The figure shows three views and two pictorial views of one solid part (mm, origin at its lowest corner). Answer the questions. A direction names the side the tool comes from. Give positions to 0.01 mm unless a question says otherwise; leave off trailing zeros. Order: outer loops, then holes, each group sorted by start corner. A loop starts at its lowest first (then second) coordinate and runs counter-clockwise, first axis right, second up. Notation, with made-up numbers: (-10, -5) - (1, -5) arc R34 ccw to (1, 29) - close; hole circle Ø11 at (39, 53). An arc over 180 degrees is marked (long way). Write item = value, one per line.
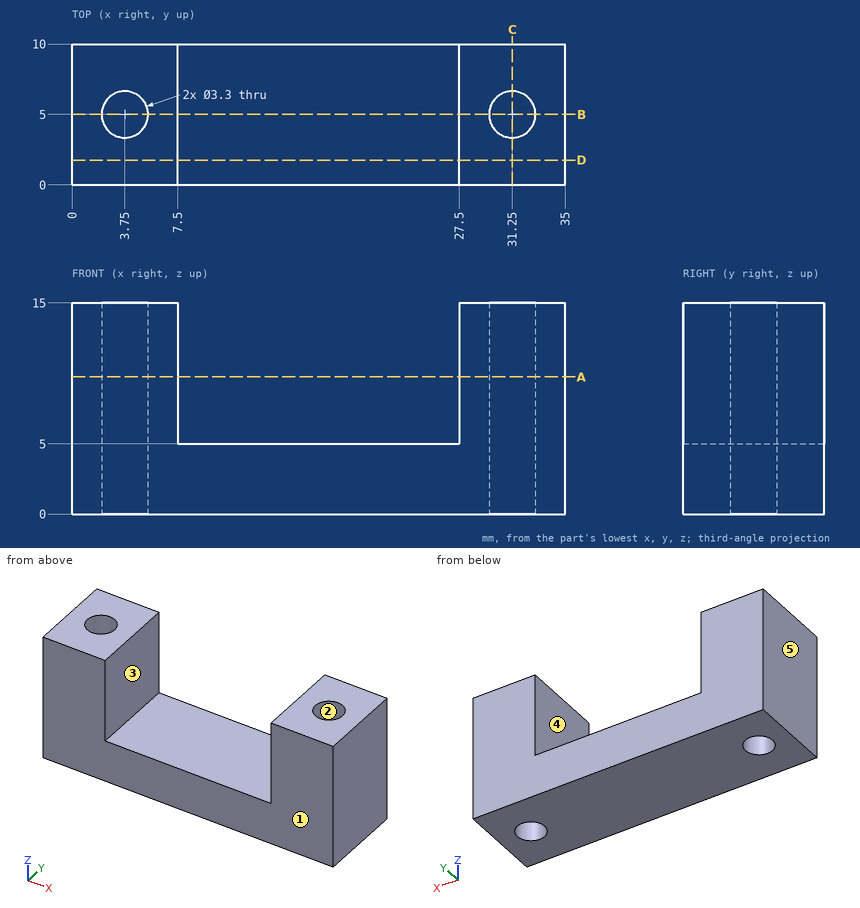
1. Determine the mould class of the marked faces 1, 2 and 3 for opening direction Y: +Y half, -Y half, draft (parallel to the pull), parting line (faces both ways), or undercut.
Recorded:
face_1 = -Y half
face_2 = undercut
face_3 = draft
2. Straight lines are drawn through the part: L1, parallel to Y at x = 31.25, z = 5.5; L2, parallel to X at y = 9, z = 9.25; L3, parallel to X at y = 5.25, z = 1.5. For each, find the intervals that lie inside material, in ascending order. Write a range as [from, to].
Recorded:
L1 = [0, 3.35], [6.65, 10]
L2 = [0, 7.5], [27.5, 35]
L3 = [0, 2.12], [5.38, 29.62], [32.88, 35]
3. For the marked faces 4 and 5, determine the directions among +Z, -Z, +X, -X, +Y, -Y from which every point of the face is accessible in a straight line to the end or side of a thin tool.
Recorded:
face_4 = +Z, +Y, -Y
face_5 = +Z, -Z, -X, +Y, -Y
4. Section B-B (y = 5) is taken. Determine the outline of the cut face in (x, z).
Recorded:
outline = (0, 0) - (2.1, 0) - (2.1, 15) - (0, 15) - close; (5.4, 0) - (29.6, 0) - (29.6, 15) - (27.5, 15) - (27.5, 5) - (7.5, 5) - (7.5, 15) - (5.4, 15) - close; (32.9, 0) - (35, 0) - (35, 15) - (32.9, 15) - close
5. Section D-D (y = 1.75) is taken. Determine the outline of the cut face in (x, z).
Recorded:
outline = (0, 0) - (35, 0) - (35, 15) - (27.5, 15) - (27.5, 5) - (7.5, 5) - (7.5, 15) - (0, 15) - close
6. Section A-A (z = 9.75) is taken. Determine the outline of the cut face in (x, y), and give its area (3 significant figures).
Recorded:
outline = (0, 0) - (7.5, 0) - (7.5, 10) - (0, 10) - close; (27.5, 0) - (35, 0) - (35, 10) - (27.5, 10) - close; hole circle Ø3.3 at (3.75, 5); hole circle Ø3.3 at (31.25, 5)
area = 133 mm^2
7. Section C-C (x = 31.25) is taken. Determine the outline of the cut face in (y, z).
Recorded:
outline = (0, 0) - (3.35, 0) - (3.35, 15) - (0, 15) - close; (6.65, 0) - (10, 0) - (10, 15) - (6.65, 15) - close
